Input: part model. Units: mm. Frame: model coordinates. A direction names the side the tool comes from. Coordinates: 2 decimals unless noted, no trailing zeros. Write each loop counter-clockwise with the first axis right and the second up, starting at its lowest first coordinate (ties: lowest second). Pieces come first, ordered by that corner, then holes. Notation, with made-up numbers: (72, -33.75) - (99, -33.75) arc R19 ccw to (99, -0.75) - close; hole circle Ø9 at (48, -19.75). An arc over 180 degrees is marked (long way). Use CSV: the item, a comma, the result in double quotes.
Autodesk Inventor part; units mm, degrees
ref_plane "Work Plane1" through (-36, -258.2, 4) normal (1, 0, 0) x (0, 0, -1)
ref_plane "YZ Plane" through (0, 0, 0) normal (1, 0, 0) x (0, 1, 0)
ref_plane "XZ Plane" through (0, 0, 0) normal (0, 1, 0) x (-1, 0, 0)
sketch "Sketch1" plane through (0, 0, 0) normal (0, 0, 1) x (1, 0, 0)
  line L0 (-101, -254.2) -> (-101, -258.2)
  line L1 (-101, -258.2) -> (-56, -258.2)
  line L2 (-56, -258.2) -> (-56, -254.2)
  line L3 (-56, -254.2) -> (-16, -254.2)
  line L4 (-16, -254.2) -> (-16, -258.2)
  line L5 (-16, -258.2) -> (29, -258.2)
  line L6 (29, -258.2) -> (29, -254.2)
  line L7 (-101, -258.2) -> (-101, -298.2)
  line L8 (29, -258.2) -> (29, -298.2)
  line L9 (29, -278.2) -> (70.7342, -278.2)
  line L10 (-56, -298.2) -> (-56, -302.2)
  line L11 (-56, -302.2) -> (-16, -302.2)
  line L12 (-16, -302.2) -> (-16, -298.2)
  line L13 (-101, -298.2) -> (-56, -298.2)
  line L14 (-16, -298.2) -> (29, -298.2)
  point P0 (0, 0)
  dimension "d0" = 40
  dimension "d1" = 40
  dimension "d2" = 130
extrude "Extrusion1" add sketch "Sketch1" along normal blind 4
sketch "Sketch2" plane through (0, 0, 4) normal (0, 0, 1) x (1, 0, 0)
  line L0 (-56, -258.2) -> (-101, -258.2)
  line L1 (-101, -258.2) -> (-101, -298.2)
  line L2 (-101, -298.2) -> (-56, -298.2)
  line L3 (-56, -298.2) -> (-56, -302.2)
  line L4 (-56, -302.2) -> (-16, -302.2)
  line L5 (-16, -302.2) -> (-16, -298.2)
  line L6 (-16, -298.2) -> (29, -298.2)
  line L7 (29, -298.2) -> (29, -258.2)
  line L8 (29, -258.2) -> (-16, -258.2)
  line L9 (-16, -258.2) -> (-16, -254.2)
  line L10 (-16, -254.2) -> (-56, -254.2)
  line L11 (-56, -254.2) -> (-56, -258.2)
  line L12 (25, -273.2) -> (29, -273.2)
  line L13 (29, -273.2) -> (29, -283.2)
  line L14 (29, -283.2) -> (25, -283.2)
  line L15 (25, -283.2) -> (25, -273.2)
  point P0 (0, 0)
  point P1 (29, -278.2)
  dimension "d5" = 4
  dimension "d6" = 10
extrude "Extrusion2" cut sketch "Sketch2" against normal blind 4 contours L7 L14 L15 L12
ref_plane "Work Plane1" through (-36, -258.2, 4) normal (1, 0, 0) x (0, 0, -1)
mirror "Mirror1" about plane through (-36, -258.2, 4) normal (1, 0, 0) of "Extrusion2"
properties part number "F4"
(1) Cut plane C-C on x = -79. Return loops of the section in (y, z), and give its area (3 significant figures).
Check values:
outline,"(-298.2, 0) - (-258.2, 0) - (-258.2, 4) - (-298.2, 4) - close"
area,"160 mm^2"
(2) Cut plane B-B on y = -277. Return loops of the section in (x, z).
Check values:
outline,"(-97, 0) - (25, 0) - (25, 4) - (-97, 4) - close"
(3) Reachability of faces 5 (the flat face through (25, -278, 2)), 6 (the flat face through (-79, -258.2, 2)), 7 (the flat face through (-16, -300, 2)), 8 (the flat face through (-56, -300, 2)) from +Z, -Z, +X, -X, +Y, -Y: full face, straight path, thin tool, end or side. Return the list, or none.
Check values:
face 5,"+Z, -Z, +X"
face 6,"+Z, -Z, -X, +Y"
face 7,"+Z, -Z, +X, -Y"
face 8,"+Z, -Z, -X, -Y"
(4) Draft query along Y for faces 1 (the flat face through (6, -298.2, 2)), 2 (the flat face through (-97, -278, 2)), 3 (the flat face through (-99, -283.2, 2)), 4 (the flat face through (-16, -256, 2)). Return one class per face: pulls with the +Y half, pulls with the -Y half, needs draft (parallel to the pull), parting line crosses it, or undercut.
Check values:
face 1,"pulls with the -Y half"
face 2,"undercut"
face 3,"undercut"
face 4,"needs draft"
(5) Pin query (flat end, axial travel): pin 1 Ø1.2 at (y, z) = (-300.5, 2.5) entering from -X; pin 2 Ø1.2 at (y, z) = (-257, 3) entering from +X; pin 3 Ø2 at (y, z) = (-276, 2.5) entering from +X. Return the tip coordinate at first contact, or that it passes through.
Check values:
pin 1,"x = -56"
pin 2,"x = -16"
pin 3,"x = 25"
(6) Cut plane A-A on z = 2.9. Return loops of the section in (x, y).
Check values:
outline,"(-101, -298.2) - (-56, -298.2) - (-56, -302.2) - (-16, -302.2) - (-16, -298.2) - (29, -298.2) - (29, -283.2) - (25, -283.2) - (25, -273.2) - (29, -273.2) - (29, -258.2) - (-16, -258.2) - (-16, -254.2) - (-56, -254.2) - (-56, -258.2) - (-101, -258.2) - (-101, -273.2) - (-97, -273.2) - (-97, -283.2) - (-101, -283.2) - close"
(7) Ray query, probe 1 along Y at (x, z) = (-89, 1.1); probe 2 along X at (y, z) = (-280, 3.4); probe 3 along X at (y, z) = (-256.5, 1.25). Return the intervals inside material, ascending. Write a range as from..to.
Check values:
probe 1,"-298.2..-258.2"
probe 2,"-97..25"
probe 3,"-56..-16"
